from build123d import *

# Parameters (mm, degrees)
ESQUISSE2_R             = 1.15
ENL_V_MAT_EXTRU_1_DEPTH = 86.212939158
ESQUISSE3_R             = 1.15
ENL_V_MAT_EXTRU_2_DEPTH = 5


with BuildPart() as part:
    # Esquisse1 → Révolution1 (revolve)
    with BuildSketch(Plane.XY, mode=Mode.PRIVATE) as r_volution1_sk:
        Polygon((0, 44.25), (27, 44.25), (27, 47.55), (24.7, 47.55), (24.7, 50.55), (27, 50.55), (27, 57.15), (21, 57.15), (21, 50.25), (18.4, 50.25), (18.4, 47.75), (13.6, 47.75), (13.6, 50.25), (10.5, 50.25), (10.5, 47.75), (5.6, 47.75), (5.6, 50.25), (0, 50.25), align=None)
    revolve(r_volution1_sk.sketch.rotate(Axis((0, 0, 0), (1, 0, 0)), 90), axis=Axis((0, 0, 0), (1, 0, 0)))

    # Esquisse2 → Enlèv. mat.-Extru.1 (cut, through all)
    with BuildSketch(Plane(origin=(27, 0, 0), x_dir=(0, 0, -1), z_dir=(1, 0, 0))):
        with Locations((0, 53.85)):
            Circle(ESQUISSE2_R)
        with Locations((46.635467994, 26.925)):
            Circle(ESQUISSE2_R)
        with Locations((46.635467994, -26.925)):
            Circle(ESQUISSE2_R)
        with Locations((0, -53.85)):
            Circle(ESQUISSE2_R)
        with Locations((-46.635467994, -26.925)):
            Circle(ESQUISSE2_R)
        with Locations((-46.635467994, 26.925)):
            Circle(ESQUISSE2_R)
    extrude(amount=-ENL_V_MAT_EXTRU_1_DEPTH, mode=Mode.SUBTRACT)

    # Esquisse3 → Enlèv. mat.-Extru.2 (cut)
    with BuildSketch(Plane.ZY):
        with Locations((0, -47)):
            Circle(ESQUISSE3_R)
        with Locations((-47, 0)):
            Circle(ESQUISSE3_R)
        with Locations((0, 47)):
            Circle(ESQUISSE3_R)
        with Locations((47, 0)):
            Circle(ESQUISSE3_R)
    extrude(amount=-ENL_V_MAT_EXTRU_2_DEPTH, mode=Mode.SUBTRACT)


solid = part.part
Build history of the part. All positions in model axes, mm. A direction names the side the tool comes from. Give positions to 0.01 mm unless a question says otherwise; leave off trailing zeros. Loops run counter-clockwise (first coordinate to the right, second up) from the corner with the lowest first, then second, coordinate; pieces in that order, holes last. Notation, with made-up numbers: (-37, 65.25) -> (17, 65.25) arc R23 ccw to (17, 93.25) -> close; hole circle Ø2 at (63, 15.25). An arc over 180 degrees is marked (long way). Answer in a Markdown table with one row per item.
Item 1: Mould opens along Y. For faces 6 (the flat face through (18.4, 44.4, 18.4)), 7 (the cylindrical face through (23.958, -2.513, -57.095)), 8 (the cylindrical face through (13.689, 39.257, 20.419)) say: pulls with the +Y half, pulls with the -Y half, needs draft (parallel to the pull), parting line crosses it, or undercut.
Findings below:
| item | result |
|---|---|
| face 6 | needs draft |
| face 7 | parting line crosses it |
| face 8 | undercut |
Item 2: Slice it at B-B on x = 16.25. Write the cut outline in (y, z).
Findings below:
| item | result |
|---|---|
| outline | circle Ø95.5 at (0, 0); hole circle Ø88.5 at (0, 0) |
Item 3: Tool access for faces 1 (the flat face through (21, 38, 34)), 2 (the cylindrical face through (25.834, 28.933, -37.734)), 3 (the flat face through (10.5, 44.4, 18.4)), 4 (the flat face through (27, 31.5, -31.5)), 5 (the flat face through (0, 44.4, -0.2)): list every direction of +Z, -Z, +X, -X, +Y, -Y with a clear straight run to the whole face (end or side of a thin tool).
Findings below:
| item | result |
|---|---|
| face 1 | -X |
| face 2 | +X |
| face 3 | none |
| face 4 | +Z, -Z, +X, +Y, -Y |
| face 5 | +Z, -Z, -X, +Y, -Y |
Item 4: Probe line 1 along Y through (x, z) = (24.05, 0); line 2 along Y through (x, z) = (26, 2) (3 decimals); line 3 along Z through (x, y) = (25.75, -18). List the from-to ranges inside material, lowest first. Write a range as [from, to].
Findings below:
| item | result |
|---|---|
| line 1 | y = [-57.15, -55], [-52.7, -44.25], [44.25, 52.7], [55, 57.15] |
| line 2 | y = [-57.115, -50.51], [-47.508, -44.205], [44.205, 47.508], [50.51, 57.115] |
| line 3 | z = [-54.24, -47.24], [-44.01, -40.42], [40.42, 44.01], [47.24, 54.24] |
Item 5: Slice it at A-A on x = 22.75. Write the cut outline in (y, z) (3 decimals).
Findings below:
| item | result |
|---|---|
| outline | circle Ø114.3 at (0, 0); hole circle Ø2.3 at (-53.85, 0); hole circle Ø88.5 at (0, 0); hole circle Ø2.3 at (-26.925, -46.635); hole circle Ø2.3 at (-26.925, 46.635); hole circle Ø2.3 at (26.925, -46.635); hole circle Ø2.3 at (26.925, 46.635); hole circle Ø2.3 at (53.85, 0) |
Item 6: Flat gauge pins, fed straight in: P1, Ø3, axis at x = 24, y = -11, coming from the +Z side; P2, Ø2.5, axis at y = 46.5, z = -0.5, coming from the -X side; P3, Ø3, axis at x = 5.5, z = 0, coming from the +Y side; P4, Ø8, axis at x = 13.5, y = 30, coming from the -Z side. Where does each tip first touch, or does it go through?
Findings below:
| item | result |
|---|---|
| P1 | stops at z = 56.35 |
| P2 | stops at x = 0 |
| P3 | stops at y = 50.25 |
| P4 | stops at z = -43 |
